Part model, mm, in its own coordinate system. A direction names the side the tool comes from. Round coordinates to 2 decimals unless told otherwise and drop trailing zeros. Loops run counter-clockwise (first coordinate to the right, second up) from the corner with the lowest first, then second, coordinate; pieces in that order, holes last. Notation, with made-up numbers: M -24.5,-22.5 L 8.5,-22.5 A13 ccw 8.5,0.5 Z; hole C 46,10 d11. An arc over 180 degrees is marked long. Put each result on its own line as item: value. Start each with the question number.
1) Slice it at A-A on x = 15. State how many separate pieces and enclosed holes the cut face has, then the cut area to 3 significant figures.
2) Slice it at C-C on z = 897. Give the cut face in (x, y), then the cut area to 3 significant figures.
3) Slice it at B-B on z = 242. Give the cut face in (x, y), then the cut area to 3 significant figures.
4) Which spindle directions (+Z, -Z, +X, -X, +Y, -Y) get a long thin tool onto all of the face, cutting with end or side? Do faces 1 (the flat face through (41, -9, 962)), 2 (the flat face through (-9, -9, 150)), 3 (the flat face through (54, -9, 725)), 4 (the flat face through (15, -9, 640)), 5 (the flat face through (33, -18, 507)). Say none if no direction does.
5) Probe line 1 along Z through (x, y) = (55, -3); line 2 along X through (y, z) = (-15.25, 491.5); line 3 along X through (y, z) = (-4.5, 680). List the from-to ranges inside material, lowest first.
6) Drop flat-ended pins along their axis: pin 1 Ø1 at (y, z) = (-15.5, 478) entering from +X; pin 2 Ø9 at (x, y) = (-5.5, -10.5) entering from -Z; pin 3 Ø1.5 at (y, z) = (-8.5, 367.5) entering from -X. Give the stop position or say it passes through.
```python
from build123d import *

# Parameters (mm, degrees)
F1_DEPTH = 18


with BuildPart() as f1:
    # F0 (on Front) → F1 (new body)
    with BuildSketch(Plane.XZ):
        Polygon((0, 0), (41, 0), (41, 75), (66, 75), (66, 225), (41, 225), (41, 275), (66, 275), (66, 425), (41, 425), (41, 575), (66, 575), (66, 725), (41, 725), (41, 775), (66, 775), (66, 925), (41, 925), (41, 1000), (-18, 1000), (-18, 915), (31, 915), (31, 860), (-18, 860), (-18, 850), (0, 850), (0, 840), (31, 840), (31, 785), (0, 785), (0, 725), (-18, 725), (-18, 715), (31, 715), (31, 660), (-18, 660), (-18, 650), (0, 650), (0, 640), (31, 640), (31, 585), (0, 585), (0, 425), (-18, 425), (-18, 415), (31, 415), (31, 360), (-18, 360), (-18, 350), (0, 350), (0, 340), (31, 340), (31, 285), (0, 285), (0, 225), (-18, 225), (-18, 215), (31, 215), (31, 160), (-18, 160), (-18, 150), (0, 150), (0, 140), (31, 140), (31, 85), (0, 85), align=None)
    extrude(amount=F1_DEPTH)


solid = f1.part
```
Recorded:
1. separate pieces: 9
1. enclosed holes: 0
1. area: 10,100 mm2
2. outline: M 31,-18 L 66,-18 L 66,0 L 31,0 Z
2. area: 630 mm2
3. outline: M 0,-18 L 41,-18 L 41,0 L 0,0 Z
3. area: 738 mm2
4. face 1: +Z, +X, +Y, -Y
4. face 2: -Z, -X, +Y, -Y
4. face 3: +X, +Y, -Y
4. face 4: -X, +Y, -Y
4. face 5: +Z, -Z, +X, -X, -Y
5. line 1: z = 75 to 225, 275 to 425, 575 to 725, 775 to 925
5. line 2: x = 0 to 41
5. line 3: x = 31 to 66
6. pin 1: stops at x = 41
6. pin 2: stops at z = 150
6. pin 3: stops at x = 31
